Here's how the part is built. I have some questions about the finished solid (model axes, mm). A direction names the side the tool comes from. Give positions to 0.01 mm unless a question says otherwise; leave off trailing zeros. Write each loop counter-clockwise with the first axis right and the second up, starting at its lowest first coordinate (ties: lowest second). Pieces come first, ordered by that corner, then holes. Notation, with made-up numbers: (12.5, 34) - (59.5, 34) arc R27 cw to (59.5, 51) - close; hole circle Ø8 at (32.5, 19.5). An arc over 180 degrees is marked (long way). One line per item, written item: value. Start each with the question number.
1) Imagine slicing it at B-B on z = 2. Write out the boundary of the cut face in (x, y) (3 decimals).
2) We'd pull the mould along X, two halves only. Please class faces 3 (the flat face through (12.7, 0, 5)), 4 (the flat face through (0, -3.969, 5)), 5 (the flat face through (0, -38.1, 5)): +X half, -X half, draft (parallel to the pull), parting line (faces both ways), or undercut.
3) Imagine slicing it at C-C on x = 0. Write out the boundary of the cut face in (y, z), plus the area to 3 significant figures.
4) I'm going to push a flat-ended pin straight in: P1, Ø3, axis at x = 0, y = 0, coming from the +Z side. Where does the tip first touch, or does it pass through?
5) Please list where these lines run through material, in increasing order: L1, parallel to Y at x = -4.5, z = 7.5; L2, parallel to Y at x = 0, z = 4; L3, parallel to X at y = -10.5, z = 2 (3 decimals). Write a range as [from, to].
6) Imagine slicing it at A-A on y = 6. Write out the boundary of the cut face in (x, z) (1 decimal).
7) On a 3-axis mill with a long thin cutter (end or side, diameter ignored), from which of +Z, -Z, +X, -X, +Y, -Y can I reach the whole of each face in a straight line? I mean faces 1 (the cylindrical face through (-11.251, 36.572, 5.634)), 2 (the flat face through (0, -34.131, 5)). Say none if no direction works.
from build123d import *

# Parameters (mm, degrees)
F0_W     = 25.4
F0_H     = 76.2
F0_W_2   = 19.05
F0_H_2   = 30.1625
F0_R     = 2.54
F1_DEPTH = 11.1125
F2_R     = 5.08


with BuildPart() as f1:
    # F0 (on Top) → F1 (new body)
    with BuildSketch(Plane.XY):
        Rectangle(F0_W, F0_H)
        with Locations((0, -19.05)):
            Rectangle(F0_W_2, F0_H_2, mode=Mode.SUBTRACT)
        Circle(F0_R, mode=Mode.SUBTRACT)
        with Locations((0, 19.05)):
            Rectangle(F0_W_2, F0_H_2, mode=Mode.SUBTRACT)
    extrude(amount=F1_DEPTH)

    # F2
    f2_edges = [f1.edges().sort_by_distance(p)[0] for p in [
        (12.7, -38.1, 5.55625),
        (-12.7, -38.1, 5.55625),
        (12.7, 38.1, 5.55625),
        (-12.7, 38.1, 5.55625),
    ]]
    fillet(f2_edges, radius=F2_R)


solid = f1.part
Numbers:
1. outline: (-12.7, -33.02) arc R5.08 ccw to (-7.62, -38.1) - (7.62, -38.1) arc R5.08 ccw to (12.7, -33.02) - (12.7, 33.02) arc R5.08 ccw to (7.62, 38.1) - (-7.62, 38.1) arc R5.08 ccw to (-12.7, 33.02) - close; hole (-9.525, -34.131) - (9.525, -34.131) - (9.525, -3.969) - (-9.525, -3.969) - close; hole (-9.525, 3.969) - (9.525, 3.969) - (9.525, 34.131) - (-9.525, 34.131) - close; hole circle Ø5.08 at (0, 0)
2. face 3: +X half
2. face 4: undercut
2. face 5: draft
3. outline: (-38.1, 0) - (-34.13, 0) - (-34.13, 11.11) - (-38.1, 11.11) - close; (-3.97, 0) - (-2.54, 0) - (-2.54, 11.11) - (-3.97, 11.11) - close; (2.54, 0) - (3.97, 0) - (3.97, 11.11) - (2.54, 11.11) - close; (34.13, 0) - (38.1, 0) - (38.1, 11.11) - (34.13, 11.11) - close
3. area: 120 mm^2
4. P1: through
5. L1: [-38.1, -34.13], [-3.97, 3.97], [34.13, 38.1]
5. L2: [-38.1, -34.13], [-3.97, -2.54], [2.54, 3.97], [34.13, 38.1]
5. L3: [-12.7, -9.525], [9.525, 12.7]
6. outline: (-12.7, 0) - (-9.5, 0) - (-9.5, 11.1) - (-12.7, 11.1) - close; (9.5, 0) - (12.7, 0) - (12.7, 11.1) - (9.5, 11.1) - close
7. face 1: +Z, -Z, -X, +Y
7. face 2: +Z, -Z
